Here's how the part is built. I have some questions about the finished solid (model axes, mm). A direction names the side the tool comes from. Give positions to 0.01 mm unless a question says otherwise; leave off trailing zeros. Order: outer loops, then holes, each group sorted by start corner. A loop starts at its lowest first (then second) coordinate and runs counter-clockwise, first axis right, second up. Notation, with made-up numbers: (-39.5, -30.5) -> (1.5, -30.5) arc R7 ccw to (1.5, -22.5) -> close; hole circle Ø4 at (74, 78). An arc over 180 degrees is marked (long way). Write each question's results on one line, items separated by ' | '. Start each with the question number.
Q1. I need wall thicknesses on line 1 along Z through (x, y) = (2.5, 5.3); line 2 along X through (y, z) = (0.7, 0); line 3 along Z through (x, y) = (0, 1). Which ranges of each line are inside material? Lowest first, please. Write a range as [from, to].
Q2. Imagine slicing it at D-D, the plane x = 10. Please give me the cut outline in (y, z), then the cut area to 3 significant figures.
Q3. Imagine slicing it at C-C, the plane z = 0. Please give me the cut outline in (x, y), then the cut area to 3 significant figures.
Q4. Imagine slicing it at B-B, the plane y = 3.85. Please give me the cut outline in (x, z), then the cut area to 3 significant figures.
Q5. Imagine slicing it at A-A, the plane x = 0. Please give me the cut outline in (y, z), then the cut area to 3 significant figures.
Q6. Thinking about a two-plate mould opening in Z: for faces 3 (the face through (0, 3, 12)), 4 (the face through (0, 4, -10)), 5 (the face through (0, 3, -12)), which applies, pulls with the +Z half, pulls with the -Z half, needs draft (parallel to the pull), parting line crosses it, or undercut?
Q7. For faces 1 (the face through (-0.2, 6, 10.5)), 2 (the face through (-12, 4, 0)), which set-ups out of +Z, -Z, +X, -X, +Y, -Y let a thin tool reach every point of the face, with its end or its side?
```python
from build123d import *

# Parameters (mm, degrees)
SKETCH1_W           = 28
SKETCH1_H           = 24
SKETCH1_R           = 8.75
BOSS_EXTRUDE1_DEPTH = 2
SKETCH2_W           = 28
SKETCH2_H           = 24
SKETCH2_W_2         = 24
SKETCH2_H_2         = 20
BOSS_EXTRUDE2_DEPTH = 4


with BuildPart() as part:
    # Sketch1 → Boss-Extrude1 (new body)
    with BuildSketch(Plane(origin=(0, 0, 0), x_dir=(1, 0, 0), z_dir=(0, 1, 0))):
        Rectangle(SKETCH1_W, SKETCH1_H)
        Circle(SKETCH1_R, mode=Mode.SUBTRACT)
    extrude(amount=BOSS_EXTRUDE1_DEPTH)

    # Sketch2 → Boss-Extrude2 (add)
    with BuildSketch(Plane(origin=(0, 2, 0), x_dir=(1, 0, 0), z_dir=(0, 1, 0))):
        Rectangle(SKETCH2_W, SKETCH2_H)
        Rectangle(SKETCH2_W_2, SKETCH2_H_2, mode=Mode.SUBTRACT)
    extrude(amount=BOSS_EXTRUDE2_DEPTH)


solid = part.part
```
Geometry check:
1) line 1: [-12, -10], [10, 12] | line 2: [-14, -8.75], [8.75, 14] | line 3: [-12, -8.75], [8.75, 12]
2) outline: (0, -12) -> (6, -12) -> (6, -10) -> (2, -10) -> (2, 10) -> (6, 10) -> (6, 12) -> (0, 12) -> close | area: 64.0 mm²
3) outline: (-14, 0) -> (-8.75, 0) -> (-8.75, 2) -> (-12, 2) -> (-12, 6) -> (-14, 6) -> close; (8.75, 0) -> (14, 0) -> (14, 6) -> (12, 6) -> (12, 2) -> (8.75, 2) -> close | area: 37.0 mm²
4) outline: (-14, -12) -> (14, -12) -> (14, 12) -> (-14, 12) -> close; hole (-12, -10) -> (12, -10) -> (12, 10) -> (-12, 10) -> close | area: 192 mm²
5) outline: (0, -12) -> (6, -12) -> (6, -10) -> (2, -10) -> (2, -8.75) -> (0, -8.75) -> close; (0, 8.75) -> (2, 8.75) -> (2, 10) -> (6, 10) -> (6, 12) -> (0, 12) -> close | area: 29.0 mm²
6) face 3: pulls with the +Z half | face 4: undercut | face 5: pulls with the -Z half
7) face 1: +Z, -Z, +X, -X, +Y | face 2: +Y
